The model under review builds one solid part; all positions refer to its coordinate system, in mm. A direction names the side the tool comes from. Give positions to 0.01 mm unless a question says otherwise; leave off trailing zeros. Loops run counter-clockwise (first coordinate to the right, second up) from the corner with the lowest first, then second, coordinate; pieces in that order, holes last. Notation, with made-up numbers: (57.5, 14.25) -> (65.5, 14.25) arc R24 ccw to (65.5, 38.25) -> close; hole circle Ø6 at (87, 9.25). An arc over 180 degrees is marked (long way). Write each question's results on one line, items separated by ' | '. Start each with the question number.
Q1. We need section C-C (x = 42.5). Write out the cut boundary in (y, z), plus the area to 3 significant figures.
Q2. Insertion check: pin 1 Ø5 at (x, y) = (-26.5, 8.5) entering from -Z; pin 2 Ø4 at (x, y) = (-17.5, -2.5) entering from -Z; pin 3 Ø1.6 at (x, y) = (32, 3) entering from +Z; pin 4 Ø5 at (x, z) = (26.5, 22.5) entering from -Y. Each pin has a flat end and moves straight along its axis. Give the tip position at first contact, or say it passes through.
Q3. We need section B-B (x = -58.5). Write out the cut boundary in (y, z).
Q4. Wall thickness on L1, parallel to Z at x = 20, y = -7; L2, parallel to Z at x = 11, y = 1; L3, parallel to Y at x = 26.5, z = 19.25: over which ranges is each line inside the solid? List them lowest first. Write a range as [from, to].
Q5. Machinability: for faces 4 (the face through (27.597, 9.209, 25.548)), 5 (the face through (-28, 0, 24.044)), which of the approach directions +Z, -Z, +X, -X, +Y, -Y give a long, thin tool a straight path to every point of the face, cutting with its end or side? Answer none if there is none.
Q6. We need section D-D (x = 8). Write out the cut boundary in (y, z), plus the area to 3 significant figures.
Q7. We need section A-A (z = 25.25). Give the number of separate pieces and of enclosed holes in the cut face, plus the area to 3 significant figures.
Q8. Mouldability with a two-part tool opening along X and no side actions: class faces 1 (the face through (69.056, 0, 21)), 2 (the face through (47.612, -9.209, 25.548)), 3 (the face through (-31.87, 0.15, 18.4)) as released by +X, released by -X, zero draft, split by the parting line, or undercut.
from build123d import *

# Parameters (mm, degrees)
F1_DEPTH  = 69.05625
F4_ANGLE  = 90
F5_W      = 5.2284544853
F5_H      = 7.121348225
F6_DEPTH  = 12.7
F7_W      = 52.8066
F7_H      = 18.3185085185
F7_H_2    = 5.8928
F9_DEPTH  = 25.4
F10_ANGLE = 350
F12_R     = 4.445
F14_DEPTH = 1.5875


# Not quite as in the source:
# - a feature names something its author has since deleted; it is built from what else it names


with BuildPart() as f1:
    # F0 (on Right) → F1 (new body, symmetric)
    with BuildSketch(Plane.YZ):
        with BuildLine():
            ThreePointArc((15.8326655208, 0), (15.688324924, -3.8842128409), (15.2560993298, -7.747))
            Line((15.2560993298, -7.747), (21.1488993298, -7.747))
            Line((21.1488993298, -7.747), (24.0952993298, -10.6299))
            Line((24.0952993298, -10.6299), (27.0416993298, -7.747))
            Line((27.0416993298, -7.747), (27.0416993298, 0))
            Line((27.0416993298, 0), (15.8326655208, 0))
        make_face()
    extrude(amount=F1_DEPTH, both=True)

    # F2: F1 across plane


with BuildPart() as f1_1:
    add(f1.part)
    add(f1.part.mirror(Plane.XY))


with BuildPart() as f1_2:
    # F4: moved
    add(f1_1.part.rotate(Axis((39.1787812114, 0, 0), (1, 0, 0)), F4_ANGLE))

    # F5 (on Front) → F6 (cut, symmetric)
    with BuildSketch(Plane.XZ):
        with Locations((-47.4936227574, 27.6051734423)):
            Rectangle(F5_W, F5_H)
        with Locations((-37.4860227574, 27.6051734423)):
            Rectangle(F5_W, F5_H)
        with Locations((-27.4784227574, 27.6051734423)):
            Rectangle(F5_W, F5_H)
        with Locations((22.5595772426, 27.6051734423)):
            Rectangle(F5_W, F5_H)
        with Locations((32.5671772426, 27.6051734423)):
            Rectangle(F5_W, F5_H)
        with Locations((42.5747772426, 27.6051734423)):
            Rectangle(F5_W, F5_H)
        with Locations((52.5823772426, 27.6051734423)):
            Rectangle(F5_W, F5_H)
    extrude(amount=F6_DEPTH, both=True, mode=Mode.SUBTRACT)


with BuildPart() as f9:
    # F7 (on face) → F9 (new body)
    with BuildSketch(Plane.XZ.offset(7.747)):
        with Locations((-6.73735, 6.0968450705)):
            Rectangle(F7_W, F7_H)
        with Locations((-6.73735, 18.2024993298)):
            Rectangle(F7_W, F7_H_2)
    extrude(amount=-F9_DEPTH)


with BuildPart() as f9_1:
    # F10: moved
    add(f9.part.rotate(Axis((-6.73735, -7.747, 21.1488993298), (1, 0, 0)), F10_ANGLE))


with BuildPart() as f1_3:
    add(f1_2.part)

    # F11: cut F9
    add(f9_1.part, mode=Mode.SUBTRACT)

    # F12
    f12_edges = [f1_3.edges().sort_by_distance(p)[0] for p in [
        (-33.14065, 0, 19.782894),
        (19.66595, 0, 19.782894),
    ]]
    fillet(f12_edges, radius=F12_R)

    # F13 (on face) → F14 (join)
    with BuildSketch(Plane(origin=(19.66595, 0, 0), x_dir=(0, -1, 0), z_dir=(-1, 0, 0))):
        Polygon((-7.7439094894, 15.2560993298), (7.747, 15.2560993298), (7.747, 16.6353280399), (-7.7439094894, 16.5785290301), align=None)
    extrude(amount=-F14_DEPTH)


solid = f1_3.part
Output:
1) outline: (-10.58, 24.04) -> (-7.75, 21.15) -> (-7.75, 15.26) arc R52.33 cw to (7.75, 15.26) -> (7.75, 21.15) -> (10.58, 24.04) -> close | area: 138 mm2
2) pin 1: z = 18.41 | pin 2: z = 19.87 | pin 3: z = 24.04 | pin 4: y = -10.63
3) outline: (-10.63, 24.1) -> (-7.75, 21.15) -> (-7.75, 15.26) arc R52.33 cw to (7.75, 15.26) -> (7.75, 21.15) -> (10.63, 24.1) -> (7.75, 27.04) -> (-7.75, 27.04) -> close
4) L1: [15.26, 24.04] | L2: [19.61, 27.04] | L3: [-7.75, 7.75]
5) face 4: +Z, +X, -X, +Y | face 5: +Z, +Y, -Y
6) outline: (-10.63, 24.1) -> (-7.75, 21.15) -> (7.75, 18.42) -> (7.75, 21.15) -> (10.63, 24.1) -> (7.75, 27.04) -> (-7.75, 27.04) -> close | area: 129 mm2
7) separate pieces: 8 | enclosed holes: 0 | area: 1,930 mm2
8) face 1: released by +X | face 2: zero draft | face 3: undercut
